CAD build for the part. Positions are in the model's coordinates, mm. Face numbers are marked on the shaded views. A direction names the side the tool comes from. Round coordinates to 2 decimals unless told otherwise and drop trailing zeros. Write each question's results on one line, items separated by ' | '. Start each with the question number.
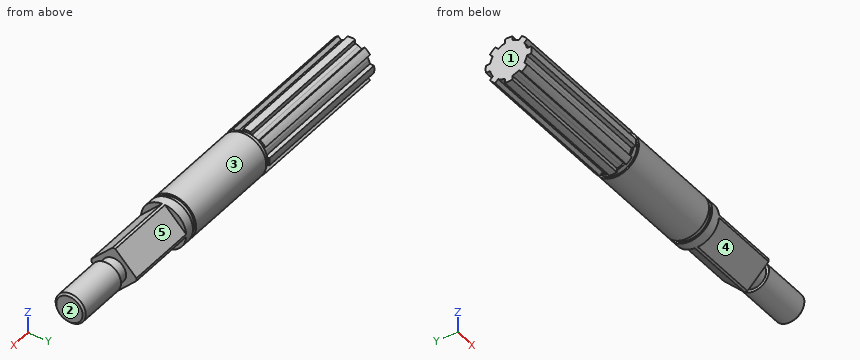
```python
from build123d import *

# Parameters (mm, degrees)
SKETCH_1_R               = 7
EXTRUDE_1_DEPTH          = 40
CUT_EXTRUDE_1_DEPTH      = 40
PATTERN_CIRCULAR_1_COUNT = 8
SKETCH_3_R               = 5.5
EXTRUDE_2_DEPTH          = 1.2
SKETCH_4_R               = 6
EXTRUDE_3_DEPTH          = 26.8
SKETCH_5_R               = 5.5
EXTRUDE_4_DEPTH          = 1.2
SKETCH_6_R               = 6
EXTRUDE_5_DEPTH          = 2.6
EXTRUDE_6_DEPTH          = 19
SKETCH_8_R               = 3.25
EXTRUDE_7_DEPTH          = 3
SKETCH_9_R               = 4
EXTRUDE_8_DEPTH          = 14
CHAMFER_1_SIZE           = 0.5
SKETCH_10_OUTSIDE_W      = 36.586
SKETCH_10_OUTSIDE_H      = 36.586
SKETCH_10_OUTSIDE_R      = 6
CUT_EXTRUDE_2_DEPTH      = 22


with BuildPart() as part:
    # Sketch 1 → Extrude 1 (new body)
    with BuildSketch(Plane(origin=(0, 0, 0), x_dir=(0, 0, -1), z_dir=(1, 0, 0))):
        Circle(SKETCH_1_R)
    extrude(amount=EXTRUDE_1_DEPTH)

    # Sketch 2 → Cut-Extrude 1 (cut)
    with BuildSketch(Plane(origin=(40, 0, 0), x_dir=(0, 0, -1), z_dir=(1, 0, 0))):
        with BuildLine():
            Line((1, 6), (1, 4.898979486))
            ThreePointArc((1, 4.898979486), (1.463400625, 4.78105204), (1.913417162, 4.619397663))
            Line((1.913417162, 4.619397663), (3.826834324, 9.238795325))
            ThreePointArc((3.826834324, 9.238795325), (0, 10), (-3.826834324, 9.238795325))
            Line((-3.826834324, 9.238795325), (-1.913417162, 4.619397663))
            ThreePointArc((-1.913417162, 4.619397663), (-1.463400625, 4.78105204), (-1, 4.898979486))
            Line((-1, 4.898979486), (-1, 6))
            ThreePointArc((-1, 6), (0, 6.08276253), (1, 6))
        make_face()
    cut_extrude_1 = extrude(amount=-CUT_EXTRUDE_1_DEPTH, mode=Mode.SUBTRACT)

    # Pattern Circular 1: Cut-Extrude 1 ×8 about axis
    pattern_circular_1_axis = Axis((0, 0, 0), (1, 0, 0))
    for i in range(1, PATTERN_CIRCULAR_1_COUNT):
        add(cut_extrude_1.rotate(pattern_circular_1_axis, i * 360 / PATTERN_CIRCULAR_1_COUNT), mode=Mode.SUBTRACT)

    # Sketch 3 → Extrude 2 (add)
    with BuildSketch(Plane(origin=(40, 0, 0), x_dir=(0, 0, -1), z_dir=(1, 0, 0))):
        with Locations(Location((0, 0, 0), (0, 0, 169.524318304))):
            Circle(SKETCH_3_R)
    extrude(amount=EXTRUDE_2_DEPTH)

    # Sketch 4 → Extrude 3 (add)
    with BuildSketch(Plane(origin=(41.2, 0, 0), x_dir=(0, 0, -1), z_dir=(1, 0, 0))):
        Circle(SKETCH_4_R)
    extrude(amount=EXTRUDE_3_DEPTH)

    # Sketch 5 → Extrude 4 (add)
    with BuildSketch(Plane(origin=(68, 0, 0), x_dir=(0, 0, -1), z_dir=(1, 0, 0))):
        with Locations(Location((0, 0, 0), (0, 0, 169.524318304))):
            Circle(SKETCH_5_R)
    extrude(amount=EXTRUDE_4_DEPTH)

    # Sketch 6 → Extrude 5 (add)
    with BuildSketch(Plane(origin=(69.2, 0, 0), x_dir=(0, 0, -1), z_dir=(1, 0, 0))):
        Circle(SKETCH_6_R)
    extrude(amount=EXTRUDE_5_DEPTH)

    # Sketch 7 → Extrude 6 (add)
    with BuildSketch(Plane(origin=(71.8, 0, 0), x_dir=(0, 0, -1), z_dir=(1, 0, 0))):
        Polygon((0, -6.363961031), (6.363961031, 0), (0, 6.363961031), (-6.363961031, 0), align=None)
    extrude(amount=EXTRUDE_6_DEPTH)

    # Sketch 8 → Extrude 7 (add)
    with BuildSketch(Plane(origin=(90.8, 0, 0), x_dir=(0, 0, -1), z_dir=(1, 0, 0))):
        Circle(SKETCH_8_R)
    extrude(amount=EXTRUDE_7_DEPTH)

    # Sketch 9 → Extrude 8 (add)
    with BuildSketch(Plane(origin=(93.8, 0, 0), x_dir=(0, 0, -1), z_dir=(1, 0, 0))):
        Circle(SKETCH_9_R)
    extrude(amount=EXTRUDE_8_DEPTH)

    # Chamfer 1
    chamfer_1_edges = [part.edges().sort_by_distance(p)[0] for p in [
        (107.8, 0, 4),
    ]]
    chamfer(chamfer_1_edges, length=CHAMFER_1_SIZE)

    # Sketch 10 outside → Cut-Extrude 2 (cut)
    with BuildSketch(Plane(origin=(71.8, 0, 0), x_dir=(0, 0, -1), z_dir=(1, 0, 0))):
        Rectangle(SKETCH_10_OUTSIDE_W, SKETCH_10_OUTSIDE_H)
        Circle(SKETCH_10_OUTSIDE_R, mode=Mode.SUBTRACT)
    extrude(amount=CUT_EXTRUDE_2_DEPTH, mode=Mode.SUBTRACT)


solid = part.part
```
1) 3-axis set-ups, long thin cutter, end or side, ignore diameter. For the marked faces 1, 2, 3, 4 and 5: which of +Z, -Z, +X, -X, +Y, -Y reach the whole face in a straight line?
2) Wall check: line 1 along X through (y, z) = (-4.75, 2.5); line 2 along Y through (x, z) = (21.5, -2.75); line 3 along Z through (x, y) = (71.5, 0.5). Give the ranges that are in metal, low to high. Write a range as from..to.
3) Drop flat-ended pins along their axis: pin 1 Ø1.5 at (x, y) = (95, 2.5) entering from +Z; pin 2 Ø0.9 at (y, z) = (-4, -4) entering from +X; pin 3 Ø0.5 at (y, z) = (-5.5, 0) entering from +X. Give the stop position or say it passes through.
Filled sheet:
1) face 1: +Z, -Z, -X, +Y, -Y | face 2: +Z, -Z, +X, +Y, -Y | face 3: +X | face 4: -Z, +X, -Y | face 5: +Z, +X, +Y
2) line 1: x = 40..71.8 | line 2: y = -4.18..4.18 | line 3: z = -5.98..5.98
3) pin 1: stops at z = 3.6 | pin 2: stops at x = 71.8 | pin 3: stops at x = 90.8
